from build123d import *

# Parameters (mm, degrees)
PAD_DEPTH    = 1
FILLET_R     = 0.3
SKETCH001_R  = 1.5
POCKET_DEPTH = 1.001


with BuildPart() as part:
    # Sketch → Pad (new body)
    with BuildSketch(Plane.XY):
        with BuildLine():
            Line((0, 0), (50, 0))
            ThreePointArc((50, 0), (57.071068, 2.928932), (60, 10))
            Line((60, 10), (60, 35))
            ThreePointArc((60, 35), (58.535534, 38.535534), (55, 40))
            Line((55, 40), (40, 40))
            ThreePointArc((40, 40), (31.746583, 38.195054), (25, 33.109746))
            Line((25, 33.109746), (0, 4))
            Line((0, 4), (0, 0))
        make_face()
    extrude(amount=PAD_DEPTH)

    # Fillet
    fillet_edges = [part.edges().sort_by_distance(p)[0] for p in [
        (31.746583, 38.195054, 1),
        (31.746583, 38.195054, 0),
        (47.5, 40, 1),
        (47.5, 40, 0),
        (12.5, 18.554873, 1),
        (12.5, 18.554873, 0),
    ]]
    fillet(fillet_edges, radius=FILLET_R)

    # Sketch001 → Pocket (cut, through all)
    with BuildSketch(Plane.XY.offset(1)):
        with Locations((10, 2)):
            Circle(SKETCH001_R)
        with Locations((35, 2)):
            Circle(SKETCH001_R)
    extrude(amount=-POCKET_DEPTH, mode=Mode.SUBTRACT)


solid = part.part
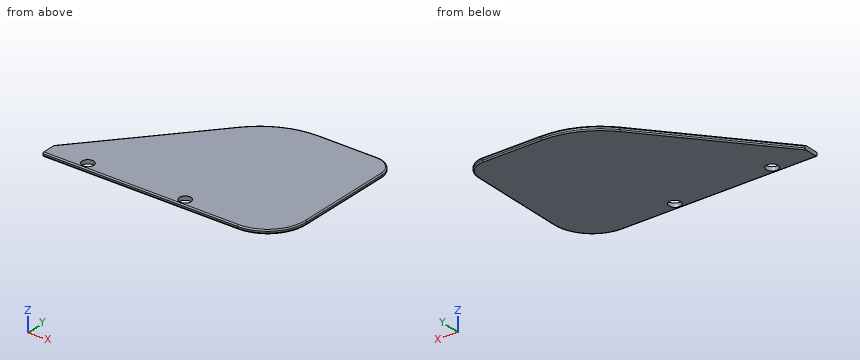
Design review of the part built by this model. Coordinates are the model's own, in mm. Round coordinates to 2 decimals unless told otherwise and drop trailing zeros. Write each loop counter-clockwise with the first axis right and the second up, starting at its lowest first coordinate (ties: lowest second). Pieces come first, ordered by that corner, then holes. Notation, with made-up numbers: (39, 44) - (60, 44) arc R21 cw to (60, 62) - close; hole circle Ø3 at (-3, -25). An arc over 180 degrees is marked (long way). Use a Markdown table: item, result. Add a question column.
1. We need section A-A (z = 0.45). State the section outline as (x, y) points, then the cut area to 3 significant figures.
2. We need section B-B (y = 2). Count the separate pieces of the cut face and the enclosed holes in it, then the cut area to 3 significant figures.
3. Wall thickness on probe 1 along Y at (x, z) = (35, 0.3); probe 2 along Y at (x, z) = (10, 0.55); probe 3 along Z at (x, y) = (9.5, 15): over which ranges is each line inside the solid? List them lowest first.
Output:
| question | item | result |
|---|---|---|
| 1 | outline | (0, 0) - (50, 0) arc R10 ccw to (60, 10) - (60, 35) arc R5 ccw to (55, 40) - (40, 40) arc R19.77 ccw to (25, 33.11) - (0, 4) - close; hole circle Ø3 at (10, 2); hole circle Ø3 at (35, 2) |
| 1 | area | 1,790 mm2 |
| 2 | separate pieces | 3 |
| 2 | enclosed holes | 0 |
| 2 | area | 49.9 mm2 |
| 3 | probe 1 | y = 0 to 0.5, 3.5 to 39.36 |
| 3 | probe 2 | y = 0 to 0.5, 3.5 to 15.64 |
| 3 | probe 3 | z = 0.15 to 0.85 |
